CAD build for the part. Positions are in the model's coordinates, mm. A direction names the side the tool comes from. Give positions to 0.01 mm unless a question says otherwise; leave off trailing zeros. Loops run counter-clockwise (first coordinate to the right, second up) from the corner with the lowest first, then second, coordinate; pieces in that order, holes last. Notation, with made-up numbers: M 19,14 L 51,14 A21 cw 51,21 Z; hole C 37,66.25 d5. An arc over 180 degrees is marked long. One line per question, with ' | ' between items.
```python
from build123d import *

# Parameters (mm, degrees)
F0_R     = 36.5
F0_R_2   = 34.5
F0_R_3   = 31.5
F0_R_4   = 22.5
F0_R_5   = 19.5
F1_DEPTH = 2
F2_DEPTH = 5
F3_R     = 1.99999
F4_R     = 2
F0_R_6   = 15.5
F5_DEPTH = 2


# Not quite as in the source:
# - a fillet or chamfer is up to 0.001 mm smaller than in the source, because OpenCascade refuses the exact size


with BuildPart() as f1:
    # F0 (on Top) → F1 (new body)
    with BuildSketch(Plane.XY):
        Circle(F0_R)
        Circle(F0_R_2, mode=Mode.SUBTRACT)
        Circle(F0_R_2)
        Circle(F0_R_3, mode=Mode.SUBTRACT)
        Circle(F0_R_3)
        Circle(F0_R_4, mode=Mode.SUBTRACT)
        Circle(F0_R_4)
        Circle(F0_R_5, mode=Mode.SUBTRACT)
    extrude(amount=F1_DEPTH)

    # F0 (on Top) → F2 (join)
    with BuildSketch(Plane.XY):
        Circle(F0_R_2)
        Circle(F0_R_3, mode=Mode.SUBTRACT)
        Circle(F0_R_4)
        Circle(F0_R_5, mode=Mode.SUBTRACT)
    extrude(amount=F2_DEPTH)

    # F3 (radius 2 in the source; OpenCascade refuses exactly that, so slightly less here)
    f3_edges = [f1.edges().sort_by_distance(p)[0] for p in [
        (-36.5, 0, 0),
    ]]
    fillet(f3_edges, radius=F3_R)

    # F4
    f4_edges = [f1.edges().sort_by_distance(p)[0] for p in [
        (-34.5, 0, 5),
    ]]
    fillet(f4_edges, radius=F4_R)

    # F0 (on Top) → F5 (join)
    with BuildSketch(Plane.XY):
        Circle(F0_R_5)
        Circle(F0_R_6, mode=Mode.SUBTRACT)
    extrude(amount=F5_DEPTH)


solid = f1.part
```
Item 1: Mould opens along Y. For faces 3 (the flat face through (-17, 27, 5)), 4 (the flat face through (-21.44, 7.44, 2)), 5 (the cylindrical face through (32.907, 10.363, 2.493)), 6 (the cylindrical face through (-4.101, 31.232, 3.479)) say: pulls with the +Y half, pulls with the -Y half, needs draft (parallel to the pull), parting line crosses it, or undercut.
Conclusion:
face 3: needs draft | face 4: undercut | face 5: parting line crosses it | face 6: undercut
Item 2: Saw through at C-C on z = 1.15. Give the cut face in (x, y).
Conclusion:
outline: C 0,0 d72.62; hole C 0,0 d31
Item 3: Drill centre lines: line 1 along Y through (x, z) = (0, 2.85); line 2 along Y through (x, z) = (0, 4.15); line 3 along X through (y, z) = (5, 2.2). Where is each one in solid material? Low to high. Write a range as [from, to].
Conclusion:
line 1: [-34.5, -31.5], [-22.5, -19.5], [19.5, 22.5], [31.5, 34.5] | line 2: [-34.14, -31.5], [-22.5, -19.5], [19.5, 22.5], [31.5, 34.14] | line 3: [-34.14, -31.1], [-21.94, -18.85], [18.85, 21.94], [31.1, 34.14]
Item 4: 3-axis set-ups, long thin cutter, end or side, ignore diameter. For faces 1 (the flat face through (-17, 10, 5)), 2 (the flat face through (-22, -27, 2)): which of +Z, -Z, +X, -X, +Y, -Y reach the whole face in a straight line?
Conclusion:
face 1: +Z, +X, -X, +Y, -Y | face 2: +Z
Item 5: Drop flat-ended pins along their axis: P1, Ø18.5, axis at x = 0, y = 0, coming from the -Z side; P2, Ø6, axis at x = 26, y = -28, coming from the +Z side. Give the stop position or say it passes through.
Conclusion:
P1: through | P2: z = 2
